The model under review builds one solid part; all positions refer to its coordinate system, in mm. A direction names the side the tool comes from. Round coordinates to 2 decimals unless told otherwise and drop trailing zeros. Loops run counter-clockwise (first coordinate to the right, second up) from the corner with the lowest first, then second, coordinate; pieces in that order, holes last. Notation, with made-up numbers: (-39, -14) -> (3, -14) arc R12 ccw to (3, -10) -> close; hole circle Ø6 at (67, 71.25). An arc over 180 degrees is marked (long way). Use a Markdown table: item, result. Add a question column.
1) Insertion check: pin 1 (1.1 mm diameter, centred on x = 8.5, y = 0.5, fed in from -Z); pin 2 (3 mm diameter, centred on y = 1, z = 15.5, fed in from +X); pin 3 (3 mm diameter, centred on y = -5.5, z = 0.5, fed in from -X); pin 4 (3 mm diameter, centred on x = 7.5, z = -19, fed in from -Y). Each pin has a flat end and moves straight along its axis. Give the tip position at first contact, or say it passes through.
2) For faces 1 (the cylindrical face through (0.179, 7.773, -31.352)), 2 (the flat face through (9, 0, 0)), 3 (the flat face through (4, 0, 17.082)), 4 (the flat face through (-9, 0, 0)), list the 3-axis set-ups (+Z, -Z, +X, -X, +Y, -Y) from which the entire face can be reached by the end or side of a thin tool; tool diameter is ignored.
3) Consider section B-B on z = -33. Give the boundary of the cut face in (x, y) (3 decimals), plus the area to 3 significant figures.
4) Wall thickness on probe 1 along Z at (x, y) = (-7.5, -1); probe 2 along Z at (x, y) = (-8.5, -0.5); probe 3 along X at (y, z) = (-5.75, -16): over which ranges is each line inside the solid? List them lowest first.
5) Mouldability with a two-part tool opening along Y and no side actions: class faces 5 (the flat face through (0, 1.52, 24)), 6 (the flat face through (7.684, 0, -12)), 7 (the cylindrical face through (0.65, -2.94, -26.03)) as released by +Y, released by -Y, zero draft, split by the parting line, or undercut.
6) Consider section A-A on y = 0. Give the boundary of the cut face in (x, z), plus the area to 3 significant figures.
7) Consider section D-D on z = -1. Give the boundary of the cut face in (x, y), plus the area to 3 significant figures.
from build123d import *

# Parameters (mm, degrees)
SKETCH1_R           = 9.9695
BOSS_EXTRUDE1_DEPTH = 17.0815
BOSS_EXTRUDE2_DEPTH = 24.9428
SKETCH3_R           = 3.5
BOSS_EXTRUDE3_DEPTH = 3
SKETCH4_R           = 1.98
BOSS_EXTRUDE4_DEPTH = 7.75
CUT_EXTRUDE1_DEPTH  = 7.1
SKETCH6_R           = 3.01
BOSS_EXTRUDE5_DEPTH = 1.8
FILLET1_R           = 0.5
FILLET2_R           = 0.1
SKETCH7_R           = 1.375
BOSS_EXTRUDE6_DEPTH = 13


with BuildPart() as part:
    # Sketch1 → Boss-Extrude1 (new body)
    with BuildSketch(Plane.XY):
        Circle(SKETCH1_R)
    extrude(amount=BOSS_EXTRUDE1_DEPTH)

    # Sketch2 → Boss-Extrude2 (add)
    with BuildSketch(Plane(origin=(0, 0, 0), x_dir=(-1, 0, 0), z_dir=(0, 0, -1))):
        with BuildLine():
            Line((-7.6835, 6.352539492), (-7.6835, -6.352539492))
            ThreePointArc((-7.6835, -6.352539492), (0, -9.9695), (7.6835, -6.352539492))
            Line((7.6835, -6.352539492), (7.6835, 6.352539492))
            ThreePointArc((7.6835, 6.352539492), (0, 9.9695), (-7.6835, 6.352539492))
        make_face()
    extrude(amount=BOSS_EXTRUDE2_DEPTH)

    # Sketch3 → Boss-Extrude3 (add)
    with BuildSketch(Plane.XY.offset(17.0815)):
        Circle(SKETCH3_R)
    extrude(amount=BOSS_EXTRUDE3_DEPTH)

    # Sketch4 → Boss-Extrude4 (add)
    with BuildSketch(Plane.XY.offset(20.0815)):
        Circle(SKETCH4_R)
    extrude(amount=BOSS_EXTRUDE4_DEPTH)

    # Sketch5 → Cut-Extrude1 (cut)
    with BuildSketch(Plane.XY.offset(27.8315)):
        with BuildLine():
            Line((-1.268857754, 1.52), (1.268857754, 1.52))
            ThreePointArc((1.268857754, 1.52), (0, 1.98), (-1.268857754, 1.52))
        make_face()
    extrude(amount=-CUT_EXTRUDE1_DEPTH, mode=Mode.SUBTRACT)

    # Sketch6 → Boss-Extrude5 (add)
    with BuildSketch(Plane(origin=(0, 0, -24.9428), x_dir=(-1, 0, 0), z_dir=(0, 0, -1))):
        Circle(SKETCH6_R)
    extrude(amount=BOSS_EXTRUDE5_DEPTH)

    # Fillet1
    fillet1_edges = [part.edges().sort_by_distance(p)[0] for p in [
        (3.01, 0, -24.9428),
    ]]
    fillet(fillet1_edges, radius=FILLET1_R)

    # Fillet2
    fillet2_edges = [part.edges().sort_by_distance(p)[0] for p in [
        (3.01, 0, -26.7428),
    ]]
    fillet(fillet2_edges, radius=FILLET2_R)

    # Sketch7 → Boss-Extrude6 (add)
    with BuildSketch(Plane(origin=(0, 0, -24.9428), x_dir=(-1, 0, 0), z_dir=(0, 0, -1))):
        with Locations((0, 6.41)):
            Circle(SKETCH7_R)
        with Locations((0, -6.41)):
            Circle(SKETCH7_R)
    extrude(amount=BOSS_EXTRUDE6_DEPTH)


solid = part.part
Result set:
| question | item | result |
|---|---|---|
| 1 | pin 1 | z = 0 |
| 1 | pin 2 | x = 9.97 |
| 1 | pin 3 | x = -9.13 |
| 1 | pin 4 | y = -7.96 |
| 2 | face 1 | -Z |
| 2 | face 2 | -Z, +X, +Y, -Y |
| 2 | face 3 | +Z |
| 2 | face 4 | -Z, -X, +Y, -Y |
| 3 | outline | circle Ø2.75 at (0, -6.41); circle Ø2.75 at (0, 6.41) |
| 3 | area | 11.9 mm2 |
| 4 | probe 1 | -24.94 to 17.08 |
| 4 | probe 2 | 0 to 17.08 |
| 4 | probe 3 | -7.68 to 7.68 |
| 5 | face 5 | released by +Y |
| 5 | face 6 | zero draft |
| 5 | face 7 | undercut |
| 6 | outline | (-9.97, 0) -> (-7.68, 0) -> (-7.68, -24.94) -> (-3.51, -24.94) arc R0.5 cw to (-3.01, -25.44) -> (-3.01, -26.64) arc R0.1 ccw to (-2.91, -26.74) -> (2.91, -26.74) arc R0.1 ccw to (3.01, -26.64) -> (3.01, -25.44) arc R0.5 cw to (3.51, -24.94) -> (7.68, -24.94) -> (7.68, 0) -> (9.97, 0) -> (9.97, 17.08) -> (3.5, 17.08) -> (3.5, 20.08) -> (1.98, 20.08) -> (1.98, 27.83) -> (-1.98, 27.83) -> (-1.98, 20.08) -> (-3.5, 20.08) -> (-3.5, 17.08) -> (-9.97, 17.08) -> close |
| 6 | area | 787 mm2 |
| 7 | outline | (-7.68, -6.35) arc R9.97 ccw to (7.68, -6.35) -> (7.68, 6.35) arc R9.97 ccw to (-7.68, 6.35) -> close |
| 7 | area | 273 mm2 |
